```python
from build123d import *

# Parameters (mm, degrees)
F0_R     = 42
F1_DEPTH = 6
F2_R     = 34
F3_DEPTH = 4
F4_R     = 20
F5_DEPTH = 2
F6_R     = 42
F6_R_2   = 39
F7_DEPTH = 3


with BuildPart() as f1:
    # F0 (on Front) → F1 (new body)
    with BuildSketch(Plane.XZ):
        Circle(F0_R)
    extrude(amount=-F1_DEPTH)

    # F2 (on face) → F3 (cut)
    with BuildSketch(Plane.XZ):
        Circle(F2_R)
    extrude(amount=-F3_DEPTH, mode=Mode.SUBTRACT)

    # F4 (on face) → F5 (cut)
    with BuildSketch(Plane.XZ.offset(-4)):
        Circle(F4_R)
    extrude(amount=-F5_DEPTH, mode=Mode.SUBTRACT)

    # F6 (on face) → F7 (cut)
    with BuildSketch(Plane.XZ):
        Circle(F6_R)
        Circle(F6_R_2, mode=Mode.SUBTRACT)
    extrude(amount=-F7_DEPTH, mode=Mode.SUBTRACT)


solid = f1.part
```
Verification items for the finished model (mm, model axes). A direction names the side the tool comes from. Coordinates: 2 decimals unless noted, no trailing zeros. Loops run counter-clockwise (first coordinate to the right, second up) from the corner with the lowest first, then second, coordinate; pieces in that order, holes last. Notation, with made-up numbers: (47.25, 41) -> (94.25, 41) arc R16 cw to (94.25, 66) -> close; hole circle Ø6 at (-21, -10.75). An arc over 180 degrees is marked (long way). Put each result on its own line as item: value.
1. Section check C-C, the plane z = -26.5. Record the boundary of the cut face in (x, y), then the cut area to 3 significant figures.
Result set:
outline: (-32.58, 3) -> (-28.61, 3) -> (-28.61, 0) -> (-21.3, 0) -> (-21.3, 4) -> (21.3, 4) -> (21.3, 0) -> (28.61, 0) -> (28.61, 3) -> (32.58, 3) -> (32.58, 6) -> (-32.58, 6) -> close
area: 197 mm^2
2. Section check D-D, the plane z = 23. Record the boundary of the cut face in (x, y).
Result set:
outline: (-35.14, 3) -> (-31.5, 3) -> (-31.5, 0) -> (-25.04, 0) -> (-25.04, 4) -> (25.04, 4) -> (25.04, 0) -> (31.5, 0) -> (31.5, 3) -> (35.14, 3) -> (35.14, 6) -> (-35.14, 6) -> close
3. Section check A-A, the plane x = 0. Record the boundary of the cut face in (y, z), then the cut area to 3 significant figures.
Result set:
outline: (0, -39) -> (3, -39) -> (3, -42) -> (6, -42) -> (6, -20) -> (4, -20) -> (4, -34) -> (0, -34) -> close; (0, 34) -> (4, 34) -> (4, 20) -> (6, 20) -> (6, 42) -> (3, 42) -> (3, 39) -> (0, 39) -> close
area: 134 mm^2
4. Thickness scan on line 1 (Z direction, x = -1, y = 3.7); line 2 (Z direction, x = 0, y = 4.6); line 3 (Y direction, x = 25, z = -6). Record the ranges inside material, lowest first.
Result set:
line 1: z = -41.99 to -33.99, 33.99 to 41.99
line 2: z = -42 to -20, 20 to 42
line 3: y = 4 to 6
5. Mould release check, pull along Z, two halves, no side actions. Record for faces 3 (the face through (18.28, 1.97, 28.67)), 4 (the face through (40.06, 4.48, 12.62)), 5 (the face through (28, 3, -28)): pulls with the +Z half, pulls with the -Z half, needs draft (parallel to the pull), parting line crosses it, or undercut.
Result set:
face 3: undercut
face 4: parting line crosses it
face 5: needs draft
6. Gauge pin test, flat ends, axial feed: P1, Ø25, axis at x = -18.5, z = 7.5, coming from the -Y side; P2, Ø1.5, axis at x = 26.5, y = 4, coming from the +Z side; P3, Ø1, axis at y = 3.5, z = -17.5, coming from the -X side. Record the tip position at first contact, or that the pin passes through.
Result set:
P1: stops at y = 4
P2: stops at z = 33.18
P3: stops at x = -38.41
7. Tool access check on faces 1 (the face through (-5.077, 1.479, 38.668)), 2 (the face through (-12, 0, 32)). Record the directions out of +Z, -Z, +X, -X, +Y, -Y that give a thin tool (end or side, any length) a straight path to the whole face; none if there is none.
Result set:
face 1: -Y
face 2: +Z, -Z, +X, -X, -Y
8. Section check B-B, the plane z = 0. Record the boundary of the cut face in (x, y).
Result set:
outline: (-42, 3) -> (-39, 3) -> (-39, 0) -> (-34, 0) -> (-34, 4) -> (-20, 4) -> (-20, 6) -> (-42, 6) -> close; (20, 4) -> (34, 4) -> (34, 0) -> (39, 0) -> (39, 3) -> (42, 3) -> (42, 6) -> (20, 6) -> close
